from build123d import *

# Parameters (mm, degrees)
PAD_DEPTH       = 140
PAD001_DEPTH    = 2
SKETCH002_W     = 15
SKETCH002_H     = 2
PAD002_DEPTH    = 55
PAD003_DEPTH    = 2
PAD004_DEPTH    = 48
SKETCH006_W     = 3
SKETCH006_H     = 5
PAD005_DEPTH    = 40
SKETCH007_W     = 2
SKETCH007_H     = 3
POCKET_DEPTH    = 40
SKETCH008_W     = 3
SKETCH008_H     = 5
PAD006_DEPTH    = 40
SKETCH009_W     = 2
SKETCH009_H     = 3
POCKET001_DEPTH = 40
PAD007_DEPTH    = 73.5
POCKET002_DEPTH = 134
POCKET003_DEPTH = 48
POCKET004_DEPTH = 72


with BuildPart() as part:
    # Sketch001 → Pad (new body)
    with BuildSketch(Plane.XY):
        Polygon((1, -3), (0, -2), (0, 0), (15, 0), (15, -2), (14, -3), align=None)
    extrude(amount=PAD_DEPTH)

    # Sketch (on Face3 of Pad) → Pad001 (join)
    with BuildSketch(Plane(origin=(0, -2, 0), x_dir=(-1, 0, 0), z_dir=(0, 1, 0))):
        Polygon((-15, 42.5195242506), (-15, 17), (-27.1352549156, 33.7027454662), align=None)
    extrude(amount=PAD001_DEPTH)

    # Sketch002 (on Face13 of Pad001) → Pad002 (join)
    with BuildSketch(Plane(origin=(25.4016078463, 0, 34.9623137906), x_dir=(0.8090169944, 0, -0.5877852523), z_dir=(0.5877852523, 0, 0.8090169944))):
        with Locations((-5.3570943733, -1)):
            Rectangle(SKETCH002_W, SKETCH002_H)
    extrude(amount=PAD002_DEPTH)

    # Sketch003 (on Face15 of Pad002) → Pad003 (join)
    with BuildSketch(Plane(origin=(0, -2, 2), x_dir=(-1, 0, 0), z_dir=(0, 1, 0))):
        Polygon((-44.4634437917, 85.0154589412), (-59.4634437917, 85.0154589412), (-59.4634437917, 76.1986801568), align=None)
    extrude(amount=PAD003_DEPTH)

    # Sketch004 (on Face26 of Pad003) → Pad004 (join)
    with BuildSketch(Plane.XY.offset(39.0154589412)):
        Polygon((59.4634437917, 0), (44.4634437917, 0), (44.4634437917, -2), (45.4634437917, -3), (58.4634437917, -3), (59.4634437917, -2), align=None)
    extrude(amount=PAD004_DEPTH)

    # Sketch006 (on Face3 of Pad004) → Pad005 (join)
    with BuildSketch(Plane(origin=(40, 0, 0), x_dir=(0, -1, 0), z_dir=(-1, 0, 0))):
        with Locations((1.5, 2.5)):
            Rectangle(SKETCH006_W, SKETCH006_H)
    extrude(amount=PAD005_DEPTH)

    # Sketch007 (on Face3 of Pad005) → Pocket (cut)
    with BuildSketch(Plane(origin=(0, 0, 0), x_dir=(0, -1, 0), z_dir=(-1, 0, 0))):
        with Locations((1, 1.5)):
            Rectangle(SKETCH007_W, SKETCH007_H)
    extrude(amount=-POCKET_DEPTH, mode=Mode.SUBTRACT)

    # Sketch008 (on Face20 of Pocket) → Pad006 (join)
    with BuildSketch(Plane(origin=(40, 0, 0), x_dir=(0, -1, 0), z_dir=(-1, 0, 0))):
        with Locations((1.5, 137.5)):
            Rectangle(SKETCH008_W, SKETCH008_H)
    extrude(amount=PAD006_DEPTH)

    # Sketch009 (on Face30 of Pad006) → Pocket001 (cut)
    with BuildSketch(Plane(origin=(0, 0, 0), x_dir=(0, -1, 0), z_dir=(-1, 0, 0))):
        with Locations((1, 138.5)):
            Rectangle(SKETCH009_W, SKETCH009_H)
    extrude(amount=-POCKET001_DEPTH, mode=Mode.SUBTRACT)

    # Sketch005 (on DatumPlane) → Pad007 (join)
    with BuildSketch(Plane(origin=(57.9083234174, -2, 76.0582405894), x_dir=(0, -1, 0), z_dir=(-0.5877852523, 0, -0.8090169944))):
        Polygon((0, 0), (0, 15), (1, 14), (1, 1), align=None)
    extrude(amount=PAD007_DEPTH)

    # Sketch010 (on Face8 of Pad007) → Pocket002 (cut)
    with BuildSketch(Plane(origin=(0, 0, 3), x_dir=(1, 0, 0), z_dir=(0, 0, -1))):
        Polygon((3, 0), (3, 1.5), (2.5, 1.5), (2.5, 2), (12.5, 2), (12.5, 1.5), (12, 1.5), (12, 0), align=None)
    extrude(amount=-POCKET002_DEPTH, mode=Mode.SUBTRACT)

    # Sketch011 (on Face66 of Pocket002) → Pocket003 (cut)
    with BuildSketch(Plane(origin=(0, 0, 39.0154589412), x_dir=(1, 0, 0), z_dir=(0, 0, -1))):
        Polygon((46.9634437917, 2), (56.9634437917, 2), (56.9634437917, 1.5), (56.4634437917, 1.5), (56.4634437917, 0), (47.4634437917, 0), (47.4634437917, 1.5), (46.9634437917, 1.5), align=None)
    extrude(amount=-POCKET003_DEPTH, mode=Mode.SUBTRACT)

    # Sketch012 (on DatumPlane) → Pocket004 (cut)
    with BuildSketch(Plane(origin=(15, -2, 17), x_dir=(0, -1, 0), z_dir=(-0.5877852523, 0, -0.8090169944))):
        Polygon((0, 2.5), (-0.5, 2.5), (-0.5, 3), (-2, 3), (-2, 12), (-0.5, 12), (-0.5, 12.5), (0, 12.5), align=None)
    extrude(amount=-POCKET004_DEPTH, mode=Mode.SUBTRACT)


solid = part.part
Can you work these out from the model? Positions are in its coordinate system, mm. A direction names the side the tool comes from. Coordinates: 2 decimals unless noted, no trailing zeros. Write each loop counter-clockwise with the first axis right and the second up, starting at its lowest first coordinate (ties: lowest second). Pieces come first, ordered by that corner, then holes. Notation, with made-up numbers: M -5,63 L 26,63 A22 ccw 26,69 Z; hole C 45,65 d8. An arc over 180 degrees is marked long. Use one line per item in the form item = value.
Q1. If we section it at A-A (z = 132): Write out the boundary of the cut face in (x, y).
Model answer:
outline = M 0,-2 L 1,-3 L 14,-3 L 15,-2 L 15,0 L 12,0 L 12,-1.5 L 12.5,-1.5 L 12.5,-2 L 2.5,-2 L 2.5,-1.5 L 3,-1.5 L 3,0 L 0,0 Z
Q2. For P1, Ø1, axis at x = 23.5, y = -1, coming from the +Z side; P2, Ø0.9, axis at y = -2, z = 2, coming from the +X side; P3, Ø1.5, axis at x = 51.5, y = -1, coming from the +Z side, each with a flat end and sliding along its axis, tell me the tip position at first contact or that it passes through.
Model answer:
P1 = 137
P2 = 40
P3 = through
Q3. If we section it at D-D (y = -2.5): Write out the boundary of the cut face in (x, z).
Model answer:
outline = M 0,0 L 40,0 L 40,5 L 14.5,5 L 14.5,17.16 L 44.96,59.09 L 44.96,39.02 L 58.96,39.02 L 58.96,87.02 L 44.96,87.02 L 44.96,82.91 L 14.5,40.98 L 14.5,135 L 40,135 L 40,140 L 0,140 L 0,135 L 0.5,135 L 0.5,5 L 0,5 Z
Q4. If we section it at B-B (x = 31): Write out the boundary of the cut face in (y, z), then the cut area to 3 significant figures.
Model answer:
outline = M -3,0 L -2,0 L -2,3 L 0,3 L 0,5 L -3,5 Z; M -3,40.72 L -2,39.02 L 0,39.02 L 0,44.13 L -1.5,44.13 L -1.5,43.28 L -2,43.28 L -2,60.29 L -1.5,60.29 L -1.5,59.44 L 0,59.44 L 0,64.54 L -2,64.54 L -3,62.84 Z; M -3,135 L 0,135 L 0,137 L -2,137 L -2,140 L -3,140 Z
area = 61.4 mm^2
Q5. I need wall thicknesses on line 1 along X through (y, z) = (-0.35, 44.5); line 2 along Z through (x, y) = (25.5, -1.35); line 3 along Z through (x, y) = (23.5, -1.45). Which ranges of each line are inside material? Lowest first, please. Write a range as from..to.
Model answer:
line_1 = 0..3, 12..15, 16.44..20.15, 31.27..34.98, 44.46..47.46, 56.46..59.46
line_2 = 3..5, 31.45..36.56, 51.87..56.97, 135..137
line_3 = 3..5, 28.7..33.8, 49.11..54.22, 135..137
Q6. We'd pull the mould along Y, two halves only. Please class faces 1 (the flat face through (58, 0, 63)), 2 (the flat face through (29.73, -1.75, 41.53)), 3 (the flat face through (27, -1, 135)): +Y half, -Y half, draft (parallel to the pull), parting line (faces both ways), or undercut.
Model answer:
face_1 = +Y half
face_2 = undercut
face_3 = draft
Q7. If we section it at C-C (z = 71.5): Write out the boundary of the cut face in (x, y), then the cut area to 3 significant figures.
Model answer:
outline = M 0,-2 L 1,-3 L 14,-3 L 15,-2 L 15,0 L 12,0 L 12,-1.5 L 12.5,-1.5 L 12.5,-2 L 2.5,-2 L 2.5,-1.5 L 3,-1.5 L 3,0 L 0,0 Z; M 36.06,-2 L 37.29,-3 L 58.46,-3 L 59.46,-2 L 59.46,0 L 56.46,0 L 56.46,-1.5 L 56.96,-1.5 L 56.96,-2 L 39.15,-2 L 39.15,-1.5 L 39.76,-1.5 L 39.76,0 L 36.06,0 Z
area = 60.6 mm^2
Q8. For faces 4 (the flat face through (40, -2.15, 3.09)), 5 (the flat face through (30.1, -1.5, 42.5)), 6 (the flat face through (29.483, -0.74, 57.35)), which set-ups out of +Z, -Z, +X, -X, +Y, -Y let a thin tool reach every point of the face, with its end or its side?
Model answer:
face_4 = -Z, +X, +Y, -Y
face_5 = none
face_6 = +Y
